Print and shaded views of the part. All mm, measured from the part's lowest x, y and z. A direction names the side the tool comes from. Round coordinates to 2 decimals unless told otherwise and drop trailing zeros. Loops run counter-clockwise (first coordinate to the right, second up) from the corner with the lowest first, then second, coordinate; pieces in that order, holes last. Notation, with made-up numbers: (-24, -27) -> (24, -27) arc R23 cw to (24, -15) -> close; hole circle Ø4 at (89.25, -35). An arc over 180 degrees is marked (long way). Answer as CSV lines item,"result".
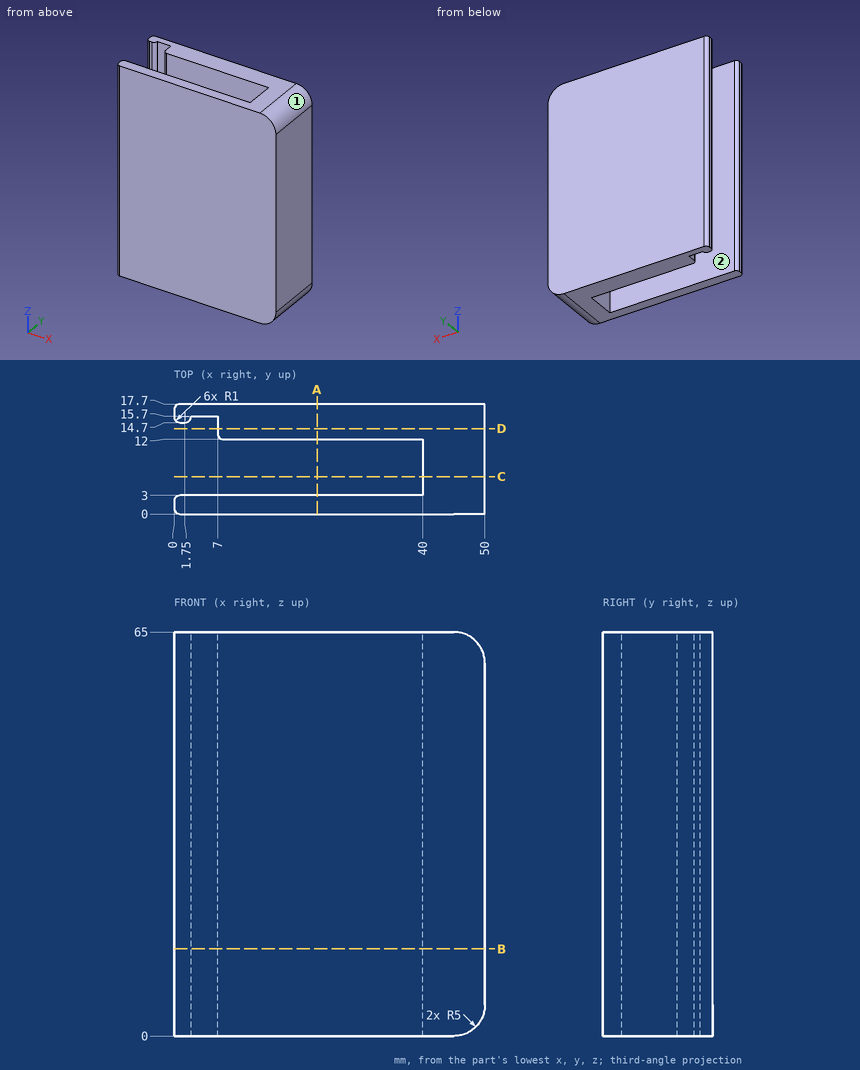
Q1. Probe L1, parallel to Y at x = 22, z = 42.5; L2, parallel to Y at x = 5.5, z = 25; L3, parallel to X at y = 5.25, z = 50.5. List the from-to ranges inside material, lowest first. Write a range as [from, to].
Results:
L1,"[0, 3], [12, 17.7]"
L2,"[0, 3], [15.7, 17.7]"
L3,"[40, 50]"
Q2. Slice it at D-D, the plane y = 13.75. Give the cut face in (x, z), and give its area (3 significant figures).
Results:
outline,"(7, 0) -> (45, 0) arc R5 ccw to (50, 5) -> (50, 60) arc R5 ccw to (45, 65) -> (7, 65) -> close"
area,"2,780 mm2"
Q3. Tool access for the marked faces 1 and 2: list every direction of +Z, -Z, +X, -X, +Y, -Y with a clear straight run to the whole face (end or side of a thin tool).
Results:
face 1,"+Z, +X, +Y, -Y"
face 2,"+Z, -Z, -X"
Q4. Slice it at A-A, the plane x = 23. Give the cut face in (y, z).
Results:
outline,"(0, 0) -> (3, 0) -> (3, 65) -> (0, 65) -> close; (12, 0) -> (17.7, 0) -> (17.7, 65) -> (12, 65) -> close"
Q5. Drop flat-ended pins along their axis: pin 1 Ø2 at (x, y) = (15, 11.5) entering from -Z; pin 2 Ø0.8 at (y, z) = (14, 23.5) entering from -X; pin 3 Ø1.5 at (y, z) = (6, 47.5) entering from -X; pin 4 Ø10 at (y, z) = (7.5, 44.5) entering from -X. Give the stop position or say it passes through.
Results:
pin 1,"z = 0"
pin 2,"x = 7"
pin 3,"x = 40"
pin 4,"x = 0.13"
Q6. Slice it at C-C, the plane y = 6. Give the cut face in (x, z).
Results:
outline,"(40, 0) -> (45, 0) arc R5 ccw to (50, 5) -> (50, 60) arc R5 ccw to (45, 65) -> (40, 65) -> close"
Q7. Slice it at B-B, the plane z = 14. Give the cut face in (x, y).
Results:
outline,"(0, 1) arc R1 ccw to (1, 0) -> (50, 0) -> (50, 17.7) -> (1, 17.7) arc R1 ccw to (0, 16.7) -> (0, 15.7) arc R1 ccw to (1, 14.7) -> (1.75, 14.7) arc R1 ccw to (2.75, 15.7) -> (7, 15.7) -> (7, 13) arc R1 ccw to (8, 12) -> (40, 12) -> (40, 3) -> (1, 3) arc R1 ccw to (0, 2) -> close"
